For this review, take the finished solid that the model builds, in its own axes (mm). Round coordinates to 2 decimals unless told otherwise and drop trailing zeros. Write each loop counter-clockwise with the first axis right and the second up, starting at its lowest first coordinate (ties: lowest second). Pieces come first, ordered by that corner, then holes. Notation, with made-up numbers: (35.5, 27.25) -> (65.5, 27.25) arc R7 cw to (65.5, 36.25) -> close; hole circle Ø11 at (79, -22). An arc over 180 degrees is marked (long way). Answer in a Markdown table with one row per item.
Autodesk Inventor part; units mm, degrees
ref_plane "YZ Plane" through (0, 0, 0) normal (1, 0, 0) x (0, 1, 0)
ref_plane "XZ Plane" through (0, 0, 0) normal (0, 1, 0) x (-1, 0, 0)
ref_plane "XY Plane" through (0, 0, 0) normal (0, 0, 1) x (1, 0, 0)
sketch "Sketch1" plane through (0, 0, 0) normal (1, 0, 0) x (0, 1, 0)
  line L0 (0, 0) -> (989.867, -571.5)
  line L1 (989.867, -571.5) -> (980.342, -587.9978)
  line L2 (980.342, -587.9978) -> (-9.525, -16.4978)
  line L3 (-9.525, -16.4978) -> (0, 0)
  line L4 (0, 0) -> (51.1145, 0)
  line L5 (980.342, -587.9978) -> (1031.142, -587.9978)
  line L6 (1031.142, -587.9978) -> (1031.142, -568.9478)
  line L7 (989.867, -571.5) -> (991.3406, -568.9478)
  line L8 (1031.142, -568.9478) -> (991.3406, -568.9478)
  line L9 (-9.525, -16.4978) -> (-7.9375, -13.7482)
  line L10 (-7.9375, -13.7482) -> (981.9295, -585.2482)
  line L11 (1031.142, -587.9978) -> (1031.142, -584.8228)
  line L12 (1031.142, -584.8228) -> (982.1751, -584.8228)
  dimension "d0" = 1143
  dimension "d1" = 19.05
  dimension "d2" = 1143
  dimension "d3" = 30
  dimension "d4" = 50.8
  dimension "d5" = 19.05
  dimension "d6" = 3.175
  dimension "d7" = 1143
  dimension "d8" = 3.175
extrude "Extrusion1" add sketch "Sketch1" along normal blind 3.175
extrude "Extrusion2" add sketch "Sketch1" against normal blind 15.875 contours L10 L1 L2 L3 | L12 L6 L5 L1
properties part number "DiagL2"
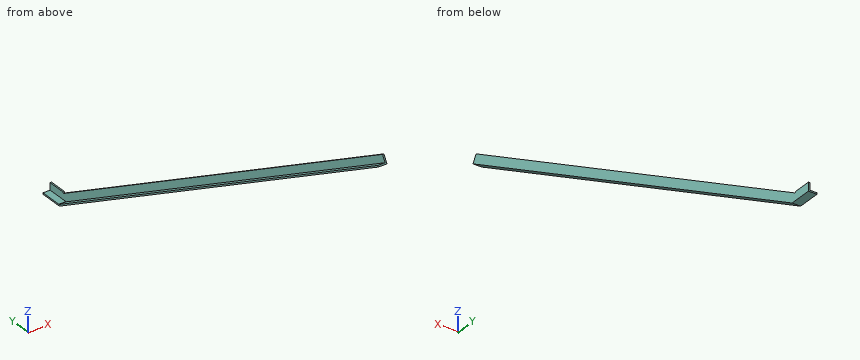
1) For line 1 (Z direction, x = -11.25, y = 532); line 2 (Y direction, x = -10.25, z = -121.5); line 3 (Z direction, x = -12.5, y = 463), list the stretches that pass through material, from the lowest coordinate up. Write a range as [from, to].
Solved:
| item | result |
|---|---|
| line 1 | [-329.15, -325.48] |
| line 2 | [172.34, 178.69] |
| line 3 | [-289.31, -285.64] |
2) Clearance check with flat-ended pins moving along their axes: pin 1 Ø1 at (x, z) = (-12.5, -402.5) entering from -Y; pin 2 Ø6 at (x, z) = (-14, -383) entering from +Y; pin 3 Ø4 at (x, z) = (1, -470) entering from -Y. State where each tip first meets the part, or that it passes through.
Solved:
| item | result |
|---|---|
| pin 1 | y = 658.18 |
| pin 2 | y = 636.82 |
| pin 3 | y = 772.5 |
3) Consider section A-A on x = -7.5. State the section outline as (y, z) points (1 decimal).
Solved:
| item | result |
|---|---|
| outline | (-9.5, -16.5) -> (980.3, -588) -> (1031.1, -588) -> (1031.1, -584.8) -> (982.2, -584.8) -> (981.9, -585.2) -> (-7.9, -13.7) -> close |
4) Consider section C-C on z = -130.5. State the section outline as (x, y) points (3 decimals), then the cut area to 3 significant figures.
Solved:
| item | result |
|---|---|
| outline | (-15.875, 187.933) -> (3.175, 187.933) -> (3.175, 226.033) -> (0, 226.033) -> (0, 194.283) -> (-15.875, 194.283) -> close |
| area | 222 mm² |
5) Consider section B-B on y = 895.5. State the section outline as (x, z) points (3 decimals), then the cut area to 3 significant figures.
Solved:
| item | result |
|---|---|
| outline | (-15.875, -539.014) -> (3.175, -539.014) -> (3.175, -517.017) -> (0, -517.017) -> (0, -535.348) -> (-15.875, -535.348) -> close |
| area | 128 mm² |
